```python
from build123d import *

# Parameters (mm, degrees)
F1_DEPTH = 25.4
F2_DEPTH = 12.7
F3_R     = 7.2804284813
F4_DEPTH = 63.5


with BuildPart() as f1:
    # F0 (on Front) → F1 (new body)
    with BuildSketch(Plane.XZ):
        Polygon((-27.2746011741, 6.805870682), (-27.2746011741, -40.3181260384), (37.7226605214, -40.3181260384), (4.2666643036, 6.805870682), align=None)
    extrude(amount=-F1_DEPTH)

    # F0 (on Front) → F2 (join)
    with BuildSketch(Plane.XZ):
        Polygon((-27.2746011741, 6.805870682), (-27.2746011741, -40.3181260384), (37.7226605214, -40.3181260384), (4.2666643036, 6.805870682), align=None)
        Polygon((4.2666643036, 6.805870682), (37.7226605214, -40.3181260384), (53.2978448683, -40.3181260384), (10.8253988259, 19.505870682), (-27.2746011741, 19.505870682), (-27.2746011741, 6.805870682), align=None)
    extrude(amount=F2_DEPTH)

    # F3 (on Right) → F4 (cut, symmetric)
    with BuildSketch(Plane.YZ):
        with Locations((12.5511875376, -16.0490572453)):
            Circle(F3_R)
    extrude(amount=F4_DEPTH, both=True, mode=Mode.SUBTRACT)


solid = f1.part
```
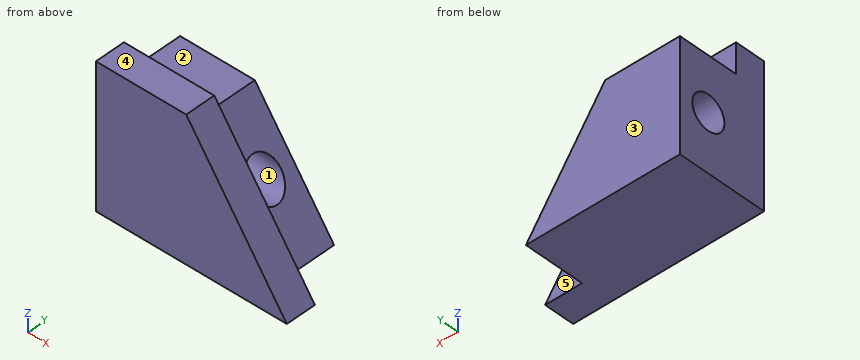
The listing builds one solid part. Answer for the finished solid, in the listing's coordinates (mm). Face numbers are marked on the shaded views. A direction names the side the tool comes from. Give positions to 0.01 mm unless a question says otherwise; leave off trailing zeros. Order: outer loops, then holes, each group sorted by start corner. A loop starts at its lowest first (then second) coordinate and runs counter-clockwise, first axis right, second up.
1) For the marked faces 4 and 5, determine the directions among +Z, -Z, +X, -X, +Y, -Y from which every point of the face is accessible in a straight line to the end or side of a thin tool.
Reported:
face 4: +Z, +X, -X, +Y, -Y
face 5: +Z, +X, +Y
2) Find section D-D on x = 7. Write down the section's boundary in (y, z), then the cut area to 3 significant figures.
Reported:
outline: (-12.7, -40.32) - (25.4, -40.32) - (25.4, 2.96) - (0, 2.96) - (0, 19.51) - (-12.7, 19.51) - close; hole circle Ø14.56 at (12.55, -16.05)
area: 1,690 mm2
3) Given P1, Ø2, axis at x = 25, y = -6.5, coming from the +Z side; P2, Ø3, axis at x = -11.5, y = 7.5, coming from the +Z side, each flat-ended and moving along its own axis, determine where each tip first touches the part or whether it passes through.
Reported:
P1: stops at z = 0.95
P2: stops at z = 6.81
4) Consider line 1 along Z through (x, y) = (-5, 12); line 2 along Z through (x, y) = (-8, 17.5); line 3 along Z through (x, y) = (-4, 24). Determine where each line is inside the solid, lowest interval first.
Reported:
line 1: z = -40.32 to -23.31, -8.79 to 6.81
line 2: z = -40.32 to -21.39, -10.71 to 6.81
line 3: z = -40.32 to 6.81
5) Find section B-B on z = -19. Write down the section's boundary in (x, y).
Reported:
outline: (-27.27, -12.7) - (38.16, -12.7) - (38.16, 0) - (22.59, 0) - (22.59, 5.9) - (-27.27, 5.9) - close; (-27.27, 19.21) - (22.59, 19.21) - (22.59, 25.4) - (-27.27, 25.4) - close
6) Determine the mould class of the marked faces 1, 2 and 3 for opening direction Y: pulls with the +Y half, pulls with the -Y half, needs draft (parallel to the pull), parting line crosses it, or undercut.
Reported:
face 1: undercut
face 2: needs draft
face 3: pulls with the +Y half
7) Find section A-A on y = 14.5. Write down the section's boundary in (x, z), then the cut area to 3 significant figures.
Reported:
outline: (-27.27, -40.32) - (37.72, -40.32) - (25.47, -23.06) - (-27.27, -23.06) - close; (-27.27, -9.03) - (15.51, -9.03) - (4.27, 6.81) - (-27.27, 6.81) - close
area: 1,600 mm2
8) Find section C-C on x = 24.5. Write down the section's boundary in (y, z), then the cut area to 3 significant figures.
Reported:
outline: (-12.7, -40.32) - (25.4, -40.32) - (25.4, -21.69) - (17.15, -21.69) arc R7.28 cw to (7.95, -21.69) - (0, -21.69) - (0, 0.24) - (-12.7, 0.24) - close
area: 978 mm2
